from build123d import *

# Parameters (mm, degrees)
SKETCH1_R                    = 4
BOSS_EXTRUDE1_DEPTH          = 0.6
EDGE_FLANGE1_STRIP_W         = 2.8
EDGE_FLANGE1_STRIP_H         = 0.6
EDGE_FLANGE1_STRIP_CUT_DEPTH = 23
EDGE_FLANGE1_DEPTH           = 23
SKETCH14_R                   = 1.5
CUT_EXTRUDE3_DEPTH           = 21.00681134
EDGE_FLANGE2_STRIP_W         = 2.8
EDGE_FLANGE2_STRIP_H         = 0.6
EDGE_FLANGE2_STRIP_CUT_DEPTH = 23
EDGE_FLANGE2_DEPTH           = 23
SKETCH13_R                   = 1.5
CUT_EXTRUDE1_DEPTH           = 29.046746692
FILLET2_R                    = 1


# Sheet-metal steps are written as plain solids
with BuildPart() as part:
    # Sketch1 → Boss-Extrude1 (new body)
    with BuildSketch(Plane.XY):
        with BuildLine():
            Line((11.5, -4), (11.5, -11.75))
            Line((11.5, -11.75), (-11.5, -11.75))
            Line((-11.5, -11.75), (-11.5, -4))
            ThreePointArc((-11.5, -4), (-7.5, 0), (-11.5, 4))
            Line((-11.5, 4), (-11.5, 11.75))
            Line((-11.5, 11.75), (11.5, 11.75))
            Line((11.5, 11.75), (11.5, 4))
            ThreePointArc((11.5, 4), (7.5, 0), (11.5, -4))
        make_face()
        Circle(SKETCH1_R, mode=Mode.SUBTRACT)
    extrude(amount=BOSS_EXTRUDE1_DEPTH)

    # Edge-Flange1 strip (across the edge) → Edge-Flange1 strip cut (cut)
    with BuildSketch(Plane(origin=(-11.5, 11.75, 0), x_dir=(0, -1, 0), z_dir=(1, 0, 0))):
        with Locations((-0.6, -0.3)):
            Rectangle(EDGE_FLANGE1_STRIP_W, EDGE_FLANGE1_STRIP_H)
    extrude(amount=EDGE_FLANGE1_STRIP_CUT_DEPTH, mode=Mode.SUBTRACT)

    # Edge-Flange1 section (across the edge) → Edge-Flange1 (add)
    with BuildSketch(Plane(origin=(-11.5, 11.75, 0), x_dir=(0, -1, 0), z_dir=(1, 0, 0))):
        with BuildLine():
            Line((0, 0.2), (0, 11.4))
            Line((0, 11.4), (0.6, 11.4))
            Line((0.6, 11.4), (0.6, 0.2))
            ThreePointArc((0.6, 0.2), (0.658578644, 0.058578644), (0.8, 0))
            Line((0.8, 0), (0.8, -0.6))
            ThreePointArc((0.8, -0.6), (0.234314575, -0.365685425), (0, 0.2))
        make_face()
    extrude(amount=EDGE_FLANGE1_DEPTH)

    # Sketch14 → Cut-Extrude3 (cut, through all)
    with BuildSketch(Plane(origin=(0, 0, 0), x_dir=(-1, 0, 0), z_dir=(0, 0, -1))):
        with Locations((-7.5, -8.75)):
            Circle(SKETCH14_R)
        with Locations((0, -8.75)):
            Circle(SKETCH14_R)
        with Locations((7.5, -8.75)):
            Circle(SKETCH14_R)
        with Locations((7.5, 8.75)):
            Circle(SKETCH14_R)
        with Locations((0, 8.75)):
            Circle(SKETCH14_R)
        with Locations((-7.5, 8.75)):
            Circle(SKETCH14_R)
    extrude(amount=-CUT_EXTRUDE3_DEPTH, mode=Mode.SUBTRACT)

    # Edge-Flange2 strip (across the edge) → Edge-Flange2 strip cut (cut)
    with BuildSketch(Plane(origin=(-11.5, -11.75, 0.6), x_dir=(0, 1, 0), z_dir=(1, 0, 0))):
        with Locations((-0.6, -0.3)):
            Rectangle(EDGE_FLANGE2_STRIP_W, EDGE_FLANGE2_STRIP_H)
    extrude(amount=EDGE_FLANGE2_STRIP_CUT_DEPTH, mode=Mode.SUBTRACT)

    # Edge-Flange2 section (across the edge) → Edge-Flange2 (add)
    with BuildSketch(Plane(origin=(-11.5, -11.75, 0.6), x_dir=(0, 1, 0), z_dir=(1, 0, 0))):
        with BuildLine():
            Line((0, 0.2), (0, 4.4))
            Line((0, 4.4), (0.6, 4.4))
            Line((0.6, 4.4), (0.6, 0.2))
            ThreePointArc((0.6, 0.2), (0.658578644, 0.058578644), (0.8, 0))
            Line((0.8, 0), (0.8, -0.6))
            ThreePointArc((0.8, -0.6), (0.234314575, -0.365685425), (0, 0.2))
        make_face()
    extrude(amount=EDGE_FLANGE2_DEPTH)

    # Sketch13 → Cut-Extrude1 (cut, through all)
    with BuildSketch(Plane.XZ.offset(-11.15)):
        with Locations(Location((7.5, -5.8, 0), (0, 0, 270))):
            Circle(SKETCH13_R)
        with Locations(Location((-7.5, -5.8, 0), (0, 0, 90))):
            Circle(SKETCH13_R)
    extrude(amount=-CUT_EXTRUDE1_DEPTH, mode=Mode.SUBTRACT)

    # Fillet2
    fillet2_edges = [part.edges().sort_by_distance(p)[0] for p in [
        (-11.5, -11.45, 5),
        (11.5, -11.45, 5),
        (-11.5, 11.45, -11.4),
        (11.5, 11.45, -11.4),
    ]]
    fillet(fillet2_edges, radius=FILLET2_R)


solid = part.part
Check sheet for the modelled part. Datum: model origin and axes. Units: mm. A direction names the side the tool comes from. Round coordinates to 2 decimals unless told otherwise and drop trailing zeros. Order: outer loops, then holes, each group sorted by start corner. A loop starts at its lowest first (then second) coordinate and runs counter-clockwise, first axis right, second up.
(1) Cross-section at A-A, the plane y = -8.75. Enter the section's corners in (x, z).
(2) Cross-section at B-B, the plane x = 0. Enter the section's corners in (y, z).
(3) Access from +Z, -Z, +X, -X, +Y, -Y to the whole of each face (thin tool, end or side, straight path). Record for faces 5 (the flat face through (0, -11.15, 3)), 6 (the flat face through (-11.5, 11.3, -3.3)).
(4) Cross-section at D-D, the plane x = -8.5. Enter the section's corners in (y, z).
(5) Draft check along X on faces 1 (the cylindrical face through (0.325, -10.214, 0.296)), 2 (the cylindrical face through (8.69, -9.66, 0.3)), 3 (the flat face through (0, -5, 0)), 4 (the cylindrical face through (-7.5, -0.1, 0.3)). Enter one of: pulls with the +X half, pulls with the -X half, needs draft (parallel to the pull), parting line crosses it, or undercut.
(6) Scan lines: probe 1 along Y at (x, z) = (0, 0.2); probe 2 along Y at (x, z) = (0, 0.35); probe 3 along Y at (x, z) = (0, 3.25). Record each from-to range of solid material in increasing order.
(7) Cross-section at C-C, the plane z = -5.8. Enter the section's corners in (x, y), and give its area (3 significant figures).
(8) Go/stop test with flat-tipped pins: P1, Ø1, axis at x = 7.5, y = 6, coming from the +Z side; P2, Ø4, axis at x = -7.5, z = -5.8, coming from the +Y side; P3, Ø2.5, axis at x = 0, y = 8.75, coming from the +Z side; P4, Ø1, axis at x = 2.5, z = 0, coming from the -Y side. Record where each tip stops, or that it passes through.
Check sheet entries:
1. outline: (-11.5, 0) - (-9, 0) - (-9, 0.6) - (-11.5, 0.6) - close; (-6, 0) - (-1.5, 0) - (-1.5, 0.6) - (-6, 0.6) - close; (1.5, 0) - (6, 0) - (6, 0.6) - (1.5, 0.6) - close; (9, 0) - (11.5, 0) - (11.5, 0.6) - (9, 0.6) - close
2. outline: (-11.75, 0.8) arc R0.8 ccw to (-10.95, 0) - (-10.25, 0) - (-10.25, 0.6) - (-10.95, 0.6) arc R0.2 cw to (-11.15, 0.8) - (-11.15, 5) - (-11.75, 5) - close; (-7.25, 0) - (-4, 0) - (-4, 0.6) - (-7.25, 0.6) - close; (4, 0) - (7.25, 0) - (7.25, 0.6) - (4, 0.6) - close; (10.25, 0) - (10.95, 0) arc R0.2 cw to (11.15, -0.2) - (11.15, -11.4) - (11.75, -11.4) - (11.75, -0.2) arc R0.8 ccw to (10.95, 0.6) - (10.25, 0.6) - close
3. face 5: +Z, +X, -X, +Y
3. face 6: +Z, -Z, -X, +Y, -Y
4. outline: (-11.75, 0.8) arc R0.8 ccw to (-10.95, 0) - (-9.87, 0) - (-9.87, 0.6) - (-10.95, 0.6) arc R0.2 cw to (-11.15, 0.8) - (-11.15, 5) - (-11.75, 5) - close; (-7.63, 0) - (-2.65, 0) - (-2.65, 0.6) - (-7.63, 0.6) - close; (2.65, 0) - (7.63, 0) - (7.63, 0.6) - (2.65, 0.6) - close; (9.87, 0) - (10.95, 0) arc R0.2 cw to (11.15, -0.2) - (11.15, -4.68) - (11.75, -4.68) - (11.75, -0.2) arc R0.8 ccw to (10.95, 0.6) - (9.87, 0.6) - close; (11.15, -11.4) - (11.75, -11.4) - (11.75, -6.92) - (11.15, -6.92) - close
5. face 1: undercut
5. face 2: undercut
5. face 3: needs draft
5. face 4: pulls with the -X half
6. probe 1: y = -11.48 to -10.25, -7.25 to -4, 4 to 7.25, 10.25 to 11.64
6. probe 2: y = -11.61 to -10.25, -7.25 to -4, 4 to 7.25, 10.25 to 11.53
6. probe 3: y = -11.75 to -11.15
7. outline: (-11.5, 11.15) - (-9, 11.15) - (-9, 11.75) - (-11.5, 11.75) - close; (-6, 11.15) - (6, 11.15) - (6, 11.75) - (-6, 11.75) - close; (9, 11.15) - (11.5, 11.15) - (11.5, 11.75) - (9, 11.75) - close
7. area: 10.2 mm2
8. P1: stops at z = 0.6
8. P2: stops at y = 11.75
8. P3: passes through
8. P4: stops at y = -11.69
